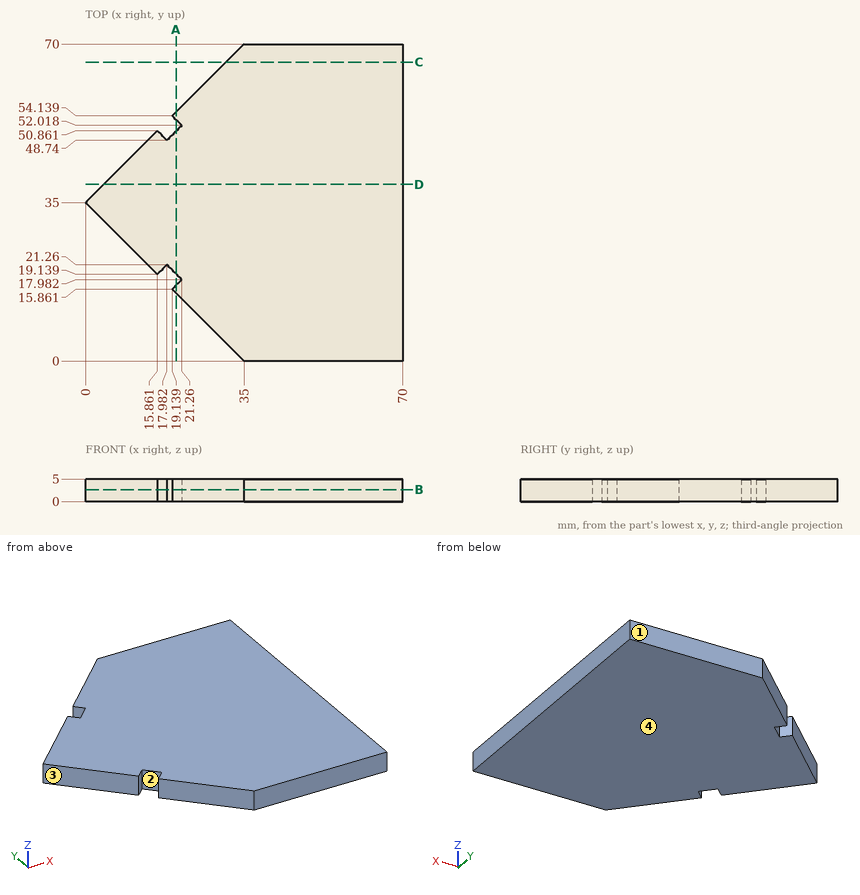
Here's the drawing with two shaded views (mm, measured from the low corner). I have some questions. Give positions to 0.01 mm unless a question says otherwise; leave off trailing zeros. Write each loop counter-clockwise with the first axis right and the second up, starting at its lowest first coordinate (ties: lowest second). Pieces come first, ordered by that corner, then holes. Notation, with made-up numbers: (76.5, -24) -> (120.5, -24) arc R14 cw to (120.5, 3) -> close; hole circle Ø3 at (55, -17). An arc over 180 degrees is marked (long way). Use one line per item in the form item = value.
1) Suppose I cut it at C-C (y = 66). Please give me the cut outline in (x, z), and give its area (3 significant figures).
Verdict:
outline = (31, 0) -> (70, 0) -> (70, 5) -> (31, 5) -> close
area = 195 mm2
2) If I drill on L1, parallel to Y at x = 20, z = 2.25 (1 decimal); L2, parallel to X at y = 30, z = 2.65; L3, parallel to X at y = 11.5, z = 4.3, over which ranges is the centre line in solid material (lowest first)? Write a range as [from, to].
Verdict:
L1 = [15, 16.7], [19.2, 50.8], [53.3, 55]
L2 = [5, 70]
L3 = [23.5, 70]
3) Suppose I cut it at A-A (x = 20). Please give me the cut outline in (y, z).
Verdict:
outline = (15, 0) -> (16.72, 0) -> (16.72, 5) -> (15, 5) -> close; (19.24, 0) -> (50.76, 0) -> (50.76, 5) -> (19.24, 5) -> close; (53.28, 0) -> (55, 0) -> (55, 5) -> (53.28, 5) -> close
4) I'm going to push a flat-ended pin straight in: pin 1 (1 mm diameter, centred on y = 13, z = 1.5, fed in from -X). Where does the tip first touch, or does it pass through?
Verdict:
pin_1 = 21.5
5) We'd pull the mould along Y, two halves only. Please class the marked faces 1, 2, 3 and 4: +Y half, -Y half, draft (parallel to the pull), parting line (faces both ways), or undercut.
Verdict:
face_1 = +Y half
face_2 = undercut
face_3 = -Y half
face_4 = draft
6) Suppose I cut it at B-B (z = 2.65). Please give me the cut outline in (x, y), and give its area (3 significant figures).
Verdict:
outline = (0, 35) -> (15.86, 19.14) -> (17.98, 21.26) -> (21.26, 17.98) -> (19.14, 15.86) -> (35, 0) -> (70, 0) -> (70, 70) -> (35, 70) -> (19.14, 54.14) -> (21.26, 52.02) -> (17.98, 48.74) -> (15.86, 50.86) -> close
area = 3,650 mm2
7) Suppose I cut it at D-D (y = 39). Please give me the cut outline in (x, z).
Verdict:
outline = (4, 0) -> (70, 0) -> (70, 5) -> (4, 5) -> close
